For this review, use the dimensioned drawing (mm, ordinates from the lowest corner) and the shaded views. A direction names the side the tool comes from. Give positions to 0.01 mm unless a question says otherwise; leave off trailing zeros. Loops run counter-clockwise (first coordinate to the right, second up) from the corner with the lowest first, then second, coordinate; pieces in that order, holes last. Notation, with made-up numbers: (74, 35.5) -> (125, 35.5) arc R17 cw to (125, 54.5) -> close; hole circle Ø2 at (-39.5, -37.5). An arc over 180 degrees is marked (long way). Use a Markdown table: item, result. Add a question column.
1. Add section B-B (z = 12.5). State the section outline as (x, y) points.
2. Add section A-A (x = 9). State the section outline as (y, z) points (1 decimal).
3. For pin 1 Ø2 at (x, y) = (16, 1.5) entering from +Z; pin 2 Ø2 at (x, y) = (16, 1.5) entering from -Z; pin 3 Ø1 at (x, y) = (25, 2.5) entering from -Z (1 decimal); pin 4 Ø5.5 at (x, z) = (7.18, 11.31) entering from -Y, all flat-tipped, find the tip position at first contact; note any pin that passes through.
4. For the marked faces 5 and 6, list the 3-axis set-ups (+Z, -Z, +X, -X, +Y, -Y) from which the entire face can be reached by the end or side of a thin tool; tool diameter is ignored.
5. Add section D-D (x = 18.5). State the section outline as (y, z) points, and give its area (3 significant figures).
6. Draft analysis for pull direction Z (two halves, no side actions). For the marked faces 1, 2, 3 and 4, state which applies: pulls with the +Z half, pulls with the -Z half, needs draft (parallel to the pull), parting line crosses it, or undercut.
7. To check wall thickness, follow line 1 (Z direction, x = 22.25, y = 0.4); line 2 (Z direction, x = 6.5, y = 2.5) (1 decimal); line 3 (X direction, y = 2.25, z = 11) (1 decimal). State the ranges of each line that lie inside material, in increasing order.
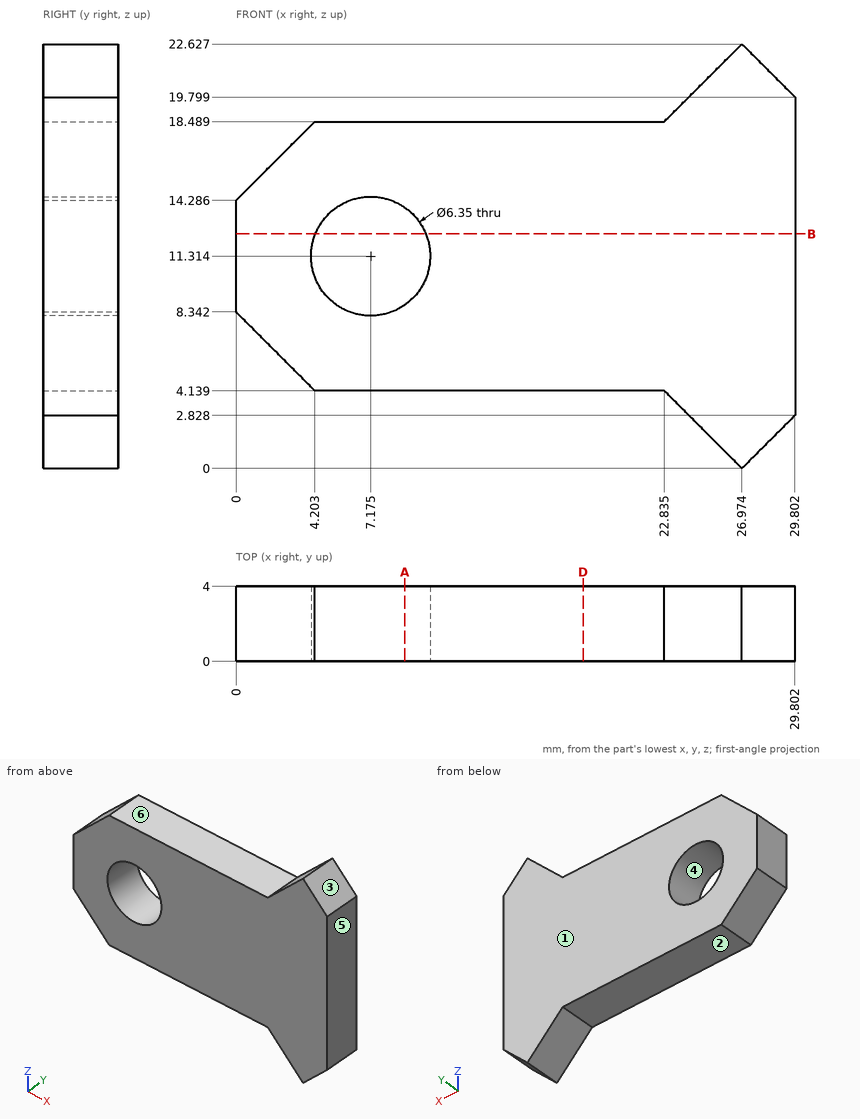
Taken from the geometry:
| question | item | result |
|---|---|---|
| 1 | outline | (0, 0) -> (4.23, 0) -> (4.23, 4) -> (0, 4) -> close; (10.12, 0) -> (29.8, 0) -> (29.8, 4) -> (10.12, 4) -> close |
| 2 | outline | (0, 4.1) -> (4, 4.1) -> (4, 8.7) -> (0, 8.7) -> close; (0, 13.9) -> (4, 13.9) -> (4, 18.5) -> (0, 18.5) -> close |
| 3 | pin 1 | stops at z = 18.49 |
| 3 | pin 2 | stops at z = 4.14 |
| 3 | pin 3 | stops at z = 1.5 |
| 3 | pin 4 | passes through |
| 4 | face 5 | +Z, -Z, +X, +Y, -Y |
| 4 | face 6 | +Z, -X, +Y, -Y |
| 5 | outline | (0, 4.14) -> (4, 4.14) -> (4, 18.49) -> (0, 18.49) -> close |
| 5 | area | 57.4 mm^2 |
| 6 | face 1 | needs draft |
| 6 | face 2 | pulls with the -Z half |
| 6 | face 3 | pulls with the +Z half |
| 6 | face 4 | undercut |
| 7 | line 1 | z = 4.14 to 18.49 |
| 7 | line 2 | z = 4.1 to 8.2, 14.4 to 18.5 |
| 7 | line 3 | x = 0 to 4, 10.3 to 29.8 |
